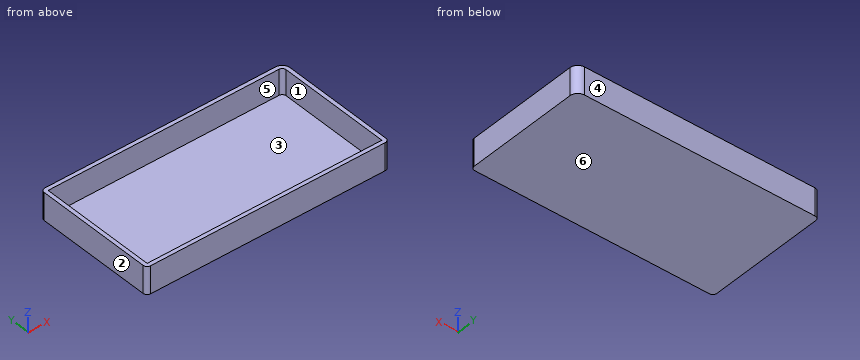
Autodesk Fusion 360 part; units mm, degrees
sketch "Sketch1" plane through (0, 0, 0) normal (0, 0, 1) x (1, 0, 0)
  line L0 (-150, 40) -> (145, 40)
  line L1 (150, 35) -> (150, -110)
  line L2 (150, -110) -> (-150, -110)
  line L3 (-150, -110) -> (-150, 40)
  arc A0 (150, 35) -> (145, 40) centre (145, 35) ccw
  line L4 (155, 35) -> (155, -110)
  line L5 (150, -115) -> (-150, -115)
  line L6 (-155, -110) -> (-155, 40)
  line L7 (-150, 45) -> (145, 45)
  arc A1 (155, 35) -> (145, 45) centre (145, 35) ccw
  arc A2 (-150, 45) -> (-155, 40) centre (-150, 40) ccw
  arc A3 (-155, -110) -> (-150, -115) centre (-150, -110) ccw
  arc A4 (150, -115) -> (155, -110) centre (150, -110) ccw
  point P0 (150, 40)
  dimension "d1" = 300
  dimension "d2" = 150
  dimension "d4" = 5
  dimension "d5" = 5
  dimension "d6" = 5
  dimension "d7" = 5
  dimension "d8" = 5
extrude "Extrude1" add sketch "Sketch1" along normal blind 20
extrude "Extrude2" add sketch "Sketch1" along normal blind 2.5 contours L0 L1 L2 L3 A0
extrude "Extrude3" add 1 faces at (50, -111.6667, 20) along direction (0, 0, 1) blind 15
Could you check a few things on this model? Use its own coordinates, in mm. Face numbers are marked on the shaded views. A direction names the side the tool comes from. Coordinates: 2 decimals unless noted, no trailing zeros. Order: outer loops, then holes, each group sorted by start corner. A loop starts at its lowest first (then second) coordinate and runs counter-clockwise, first axis right, second up. Notation, with made-up numbers: (11, 59.5) -> (28, 59.5) arc R24 ccw to (28, 81.5) -> close; hole circle Ø10 at (25, 34.25). An arc over 180 degrees is marked (long way). One line per item, written item: value. Start each with the question number.
1) Imagine slicing it at B-B on y = -3.5. List the corners of the cut face in (x, z) for me.
2) Imagine slicing it at A-A on z = 21.5. List the corners of the cut face in (x, y) for me, plus the area to 3 significant figures.
3) Imagine slicing it at C-C on x = 102.5. List the corners of the cut face in (y, z) for me, plus the area to 3 significant figures.
4) I'm going to push a flat-ended pin straight in: pin 1 (8 mm diameter, centred on x = 69, y = -18.5, fed in from +Z). Where does the tip first touch, or does it pass through?
5) Which directions (+Z, -Z, +X, -X, +Y, -Y) give clear straight access to the entire face, cutting with the end or side of a thin tool? Please do the marked faces 1 and 2.
6) If I drill on L1, parallel to Y at x = 36.5, z = 10.5; L2, parallel to X at y = -60, z = 12.5; L3, parallel to Z at x = -50, y = -28, over which ranges is the centre line in solid material (lowest first)? Write a range as [from, to].
7) We'd pull the mould along Y, two halves only. Please class the marked faces 3, 4, 5 and 6: +Y half, -Y half, draft (parallel to the pull), parting line (faces both ways), or undercut.
Answer list:
1. outline: (-155, 0) -> (155, 0) -> (155, 35) -> (150, 35) -> (150, 2.5) -> (-150, 2.5) -> (-150, 35) -> (-155, 35) -> close
2. outline: (-155, -110) arc R5 ccw to (-150, -115) -> (150, -115) arc R5 ccw to (155, -110) -> (155, 35) arc R10 ccw to (145, 45) -> (-150, 45) arc R5 ccw to (-155, 40) -> close; hole (-150, -110) -> (150, -110) -> (150, 35) arc R5 ccw to (145, 40) -> (-150, 40) -> close
2. area: 4,570 mm2
3. outline: (-115, 0) -> (45, 0) -> (45, 35) -> (40, 35) -> (40, 2.5) -> (-110, 2.5) -> (-110, 35) -> (-115, 35) -> close
3. area: 725 mm2
4. pin 1: stops at z = 2.5
5. face 1: +Z
5. face 2: +Z, -Z, -X, +Y, -Y
6. L1: y = [-115, -110], [40, 45]
6. L2: x = [-155, -150], [150, 155]
6. L3: z = [0, 2.5]
7. face 3: undercut
7. face 4: +Y half
7. face 5: undercut
7. face 6: draft
